Design review of the part built by this model. Coordinates are the model's own, in mm. A direction names the side the tool comes from. Give positions to 0.01 mm unless a question says otherwise; leave off trailing zeros. Loops run counter-clockwise (first coordinate to the right, second up) from the corner with the lowest first, then second, coordinate; pieces in that order, holes last. Notation, with made-up numbers: (75.25, 81.5) - (89.25, 81.5) arc R13 ccw to (89.25, 93.5) - close; hole circle Ø4 at (-33.5, 80). An arc over 180 degrees is marked (long way). Write each question's results on one line, items separated by ' | '.
Autodesk Inventor part; units mm, degrees
ref_plane "YZ Plane" through (0, 0, 0) normal (1, 0, 0) x (0, 1, 0)
ref_plane "XZ Plane" through (0, 0, 0) normal (0, 1, 0) x (-1, 0, 0)
ref_plane "XY Plane" through (0, 0, 0) normal (0, 0, 1) x (1, 0, 0)
sketch "Sketch1" plane through (0, 0, 0) normal (0, 0, 1) x (1, 0, 0)
  circle A0 centre (0, 0) radius 9.12
  dimension "d0" = 18.24
extrude "Extrusion1" add sketch "Sketch1" along normal blind 11.09
sketch "Sketch2" plane through (0, 0, 11.09) normal (0, 0, 1) x (1, 0, 0)
  circle A0 centre (0, 0) radius 10.285
  dimension "d3" = 20.57
extrude "Extrusion2" add sketch "Sketch2" along normal blind 9.53
sketch "Sketch3" plane through (0, 0, 20.62) normal (0, 0, 1) x (1, 0, 0)
  circle A0 centre (0, 0) radius 5.795
  dimension "d6" = 11.59
extrude "Extrusion3" cut sketch "Sketch3" against normal blind 33.78
sketch "Sketch4" plane through (0, 0, 0) normal (0, 1, 0) x (-1, 0, 0)
  line L0 (1.175, 17.44) -> (-1.175, 17.44)
  line L1 (-1.175, 17.44) -> (-1.175, 23.8)
  line L2 (-1.175, 23.8) -> (1.175, 23.8)
  line L3 (1.175, 23.8) -> (1.175, 17.44)
  line L4 (10.285, 20.62) -> (-10.285, 20.62)
  line L5 (1.175, 17.44) -> (-1.175, 23.8) construction
  line L6 (-1.175, 17.44) -> (1.175, 23.8) construction
  point P0 (0, 0)
  point P1 (0, 20.62)
  dimension "d9" = 2.35
  dimension "d10" = 6.36
extrude "Extrusion4" cut sketch "Sketch4" along normal mid plane 33.78
properties part number "parça5"
(1) Tool access review of faces 1 (the flat face through (1.175, -8, 19)), 2 (the flat face through (0, -6, 0)), 3 (the cylindrical face through (-7.237, 5.549, 5.467)): name each direction out of +Z, -Z, +X, -X, +Y, -Y from which nothing blocks a thin tool from reaching the whole face with its end or side.
Answers below:
face 1: +Z, +Y, -Y | face 2: -Z, +X, -X, +Y, -Y | face 3: -Z
(2) Take a section at A-A on y = 0. Give the boundary of the cut face in (x, z) (3 decimals), plus the area to 3 significant figures.
Answers below:
outline: (-10.285, 11.09) - (-9.12, 11.09) - (-9.12, 0) - (-5.795, 0) - (-5.795, 20.62) - (-10.285, 20.62) - close; (5.795, 0) - (9.12, 0) - (9.12, 11.09) - (10.285, 11.09) - (10.285, 20.62) - (5.795, 20.62) - close | area: 159 mm2
(3) Wall thickness on line 1 along Y through (x, z) = (0, 2.5) (3 decimals); line 2 along Y through (x, z) = (0, 11.25) (3 decimals); line 3 along X through (y, z) = (-6, 17.75) (3 decimals): over which ranges is each line inside the solid? List them lowest first. Write a range as from..to.
Answers below:
line 1: -9.12..-5.795, 5.795..9.12 | line 2: -10.285..-5.795, 5.795..10.285 | line 3: -8.354..-1.175, 1.175..8.354
(4) Insertion check: P1, Ø0.7, axis at x = 0, y = 9, coming from the +Z side; P2, Ø4, axis at y = -6, z = 3.5, coming from the +X side; P3, Ø3, axis at y = 3, z = 6, coming from the -X side; P4, Ø10.5, axis at x = 0, y = 0, coming from the +Z side. Each pin has a flat end and moves straight along its axis. Give the tip position at first contact, or say it passes through.
Answers below:
P1: z = 17.44 | P2: x = 8.2 | P3: x = -9 | P4: through
(5) Take a section at B-B on z = 18.25. Give the boundary of the cut face in (x, y) (3 decimals).
Answers below:
outline: (-1.175, -10.218) - (-1.175, -5.675) arc R5.795 cw to (-1.175, 5.675) - (-1.175, 10.218) arc R10.285 ccw to start; (1.175, -10.218) arc R10.285 ccw to (1.175, 10.218) - (1.175, 5.675) arc R5.795 cw to (1.175, -5.675) - close
(6) Take a section at C-C on x = 0.5. Give the boundary of the cut face in (y, z), plus the area to 3 significant figures.
Answers below:
outline: (-10.27, 11.09) - (-9.11, 11.09) - (-9.11, 0) - (-5.77, 0) - (-5.77, 17.44) - (-10.27, 17.44) - close; (5.77, 0) - (9.11, 0) - (9.11, 11.09) - (10.27, 11.09) - (10.27, 17.44) - (5.77, 17.44) - close | area: 131 mm2
(7) Draft analysis for pull direction X (two halves, no side actions). For faces 4 (the flat face through (-6, 0, 20.62)), 5 (the flat face through (1.175, 8, 19)), 6 (the cylindrical face through (2.674, -5.141, 10.454)), 7 (the cylindrical face through (-8.16, 6.26, 15.79)), state which applies: pulls with the +X half, pulls with the -X half, needs draft (parallel to the pull), parting line crosses it, or undercut.
Answers below:
face 4: needs draft | face 5: undercut | face 6: undercut | face 7: parting line crosses it
(8) Take a section at D-D on z = 5. Give the boundary of the cut face in (x, y) (3 decimals).
Answers below:
outline: circle Ø18.24 at (0, 0); hole circle Ø11.59 at (0, 0)
